```python
from build123d import *

# Parameters (mm, degrees)
BOSS_EXTRUDE1_DEPTH = 25.4
SKETCH2_R           = 14.2875
CUT_EXTRUDE1_DEPTH  = 83.854726027
SKETCH3_W           = 50.8
SKETCH3_H           = 38.1
CUT_EXTRUDE3_DEPTH  = 9.525
SKETCH4_W           = 11.43
SKETCH4_H           = 12.7
BOSS_EXTRUDE2_DEPTH = 38.1
CHAMFER1_SIZE       = 6.35
SKETCH5_W           = 6.35
SKETCH5_H           = 69.85
BOSS_EXTRUDE3_DEPTH = 95.25
SKETCH7_R           = 6.35
CUT_EXTRUDE5_DEPTH  = 145.139405178
SKETCH8_W           = 38.1
SKETCH8_H           = 9.525
CUT_EXTRUDE6_DEPTH  = 9.525
CHAMFER4_SIZE       = 9.525
SKETCH10_W          = 50.8
SKETCH10_H          = 72.641150816
BOSS_EXTRUDE5_DEPTH = 6.35
BOSS_EXTRUDE9_DEPTH = 50.8
SKETCH13_W          = 38.1
SKETCH13_H          = 50.8
CUT_EXTRUDE8_DEPTH  = 6.3754
SKETCH14_R          = 2.4892
CUT_EXTRUDE9_DEPTH  = 19.05
SKETCH15_R          = 2.4892
CUT_EXTRUDE10_DEPTH = 19.0246


with BuildPart() as part:
    # Sketch1 → Boss-Extrude1 (new, symmetric)
    with BuildSketch(Plane.XY):
        Polygon((-25.4, -47.625), (-19.05, -47.625), (-19.05, -9.525), (19.05, -9.525), (19.05, -47.625), (25.4, -47.625), (25.4, 60.325), (19.05, 60.325), (19.05, 9.525), (-19.05, 9.525), (-19.05, 60.325), (-25.4, 60.325), align=None)
    extrude(amount=BOSS_EXTRUDE1_DEPTH, both=True)

    # Sketch2 → Cut-Extrude1 (cut, through all)
    with BuildSketch(Plane.ZY.offset(25.4)):
        with Locations(Location((0, 34.925, 0), (0, 0, 270))):
            Circle(SKETCH2_R)
    extrude(amount=-CUT_EXTRUDE1_DEPTH, mode=Mode.SUBTRACT)

    # Sketch3 → Cut-Extrude3 (cut)
    with BuildSketch(Plane(origin=(0, 0, 25.4), x_dir=(-1, 0, 0), z_dir=(0, 0, -1))):
        with Locations((0, -28.575)):
            Rectangle(SKETCH3_W, SKETCH3_H)
    extrude(amount=CUT_EXTRUDE3_DEPTH, mode=Mode.SUBTRACT)

    # Sketch4 → Boss-Extrude2 (add)
    with BuildSketch(Plane.ZY.offset(-19.05)):
        with Locations((-19.685, 53.975)):
            Rectangle(SKETCH4_W, SKETCH4_H)
    extrude(amount=BOSS_EXTRUDE2_DEPTH)

    # Chamfer1
    chamfer1_edges = [part.edges().sort_by_distance(p)[0] for p in [
        (0, 60.325, -25.4),
    ]]
    chamfer(chamfer1_edges, length=CHAMFER1_SIZE)

    # Sketch5 → Boss-Extrude3 (add)
    with BuildSketch(Plane.XY.offset(25.4)):
        with Locations((-22.225, 25.4)):
            Rectangle(SKETCH5_W, SKETCH5_H)
        with Locations((22.225, 25.4)):
            Rectangle(SKETCH5_W, SKETCH5_H)
    extrude(amount=BOSS_EXTRUDE3_DEPTH)

    # Sketch7 → Cut-Extrude5 (cut, through all)
    with BuildSketch(Plane.ZY.offset(25.4)):
        with Locations(Location((38.1, 6.35, 0), (0, 0, 270))):
            Circle(SKETCH7_R)
    extrude(amount=-CUT_EXTRUDE5_DEPTH, mode=Mode.SUBTRACT)

    # Sketch8 → Cut-Extrude6 (cut)
    with BuildSketch(Plane.XY.offset(25.4)):
        with Locations((0, 4.7625)):
            Rectangle(SKETCH8_W, SKETCH8_H)
    extrude(amount=-CUT_EXTRUDE6_DEPTH, mode=Mode.SUBTRACT)

    # Chamfer4
    chamfer4_edges = [part.edges().sort_by_distance(p)[0] for p in [
        (0, 0, 25.4),
    ]]
    chamfer(chamfer4_edges, length=CHAMFER4_SIZE - 0.0001)  # a hair under: the kernel refuses the full size

    # Sketch10 → Boss-Extrude5 (add)
    with BuildSketch(Plane.XZ.offset(9.525)):
        with Locations((0, 84.329424592)):
            Rectangle(SKETCH10_W, SKETCH10_H)
    extrude(amount=BOSS_EXTRUDE5_DEPTH)

    # Sketch12 → Boss-Extrude9 (add)
    with BuildSketch(Plane.XY.offset(120.65)):
        Polygon((-25.4, 60.325), (-19.05, 60.325), (-19.05, 9.525), (19.05, 9.525), (19.05, 60.325), (25.4, 60.325), (25.4, -47.625), (19.05, -47.625), (19.05, -15.875), (-19.05, -15.875), (-19.05, -47.625), (-25.4, -47.625), align=None)
    extrude(amount=BOSS_EXTRUDE9_DEPTH)

    # Sketch13 → Cut-Extrude8 (cut)
    with BuildSketch(Plane(origin=(0, -15.875, 0), x_dir=(-1, 0, 0), z_dir=(0, -1, 0))):
        with Locations((0, -146.05)):
            Rectangle(SKETCH13_W, SKETCH13_H)
    extrude(amount=-CUT_EXTRUDE8_DEPTH, mode=Mode.SUBTRACT)

    # Sketch14 → Cut-Extrude9 (cut)
    with BuildSketch(Plane.XZ.offset(9.525)):
        with Locations(Location((0, -19.05, 0), (0, 0, 270))):
            Circle(SKETCH14_R)
        with Locations(Location((0, 6.35, 0), (0, 0, 270))):
            Circle(SKETCH14_R)
    extrude(amount=-CUT_EXTRUDE9_DEPTH, mode=Mode.SUBTRACT)

    # Sketch15 → Cut-Extrude10 (cut)
    with BuildSketch(Plane.XZ.offset(9.4996)):
        with Locations(Location((0, 158.75, 0), (0, 0, 270))):
            Circle(SKETCH15_R)
        with Locations(Location((0, 133.35, 0), (0, 0, 270))):
            Circle(SKETCH15_R)
    extrude(amount=-CUT_EXTRUDE10_DEPTH, mode=Mode.SUBTRACT)


solid = part.part
```
Geometry check sheet. Reference: the model listing, model coordinates, mm. A direction names the side the tool comes from. Coordinates: 2 decimals unless noted, no trailing zeros. Write each loop counter-clockwise with the first axis right and the second up, starting at its lowest first coordinate (ties: lowest second). Pieces come first, ordered by that corner, then holes. Notation, with made-up numbers: M 34.5,37 L 69.5,37 A13 cw 69.5,47 Z; hole C -15,73.5 d8. An arc over 180 degrees is marked long. Use one line per item in the form item = value. Start each with the question number.
1) Set-up check for faces 1 (the flat face through (19.05, -28, -4)), 2 (the flat face through (19.05, 19, 96)), 3 (the flat face through (0, 9.525, 146)), 4 (the flat face through (22, -32, 120.65)), 5 (the flat face through (-0.267, -4.696, 20.571)): record each of +Z, -Z, +X, -X, +Y, -Y from which the full face is reachable in a straight line by a thin tool's end or side.
2) Section check A-A on x = -12. State how many separate pieces and enclosed holes the cut face has, and give its area (3 significant figures).
3) Go/stop test with flat-tipped pins: pin 1 Ø1.9 at (x, y) = (-12.5, -14) entering from -Z; pin 2 Ø2 at (x, z) = (7.5, 139) entering from -Y. Record where each tip stops, or that it passes through.
4) Thickness scan on probe 1 along X at (y, z) = (28, 91.5); probe 2 along Y at (x, z) = (12.5, -14.5) (3 decimals); probe 3 along Z at (x, y) = (-22, 6). Record the ranges inside material, lowest first. Write a range as from..to.
5) Section check D-D on y = -19. Enter the section's corners in (x, z) (3 decimals), and give its area (3 significant figures).
6) Section check B-B on z = 133.35. Enter the section's corners in (x, y) (3 decimals).
7) Section check C-C on y = 18.5. Enter the section's corners in (x, z), and give its area (3 significant figures).
8) Release check for a two-part mould opening along Z. For faces 6 (the flat face through (-22, -28, 15.875)), 7 (the flat face through (-21, 60.325, 62)), 8 (the flat face through (0, -13, 120.65)) record: pulls with the +Z half, pulls with the -Z half, needs draft (parallel to the pull), parting line crosses it, or undercut.
Responses:
q1.face_1 = -Z, -Y
q1.face_2 = none
q1.face_3 = +Z, -Z, +Y
q1.face_4 = +X, -X, -Y
q1.face_5 = +Y
q2.separate_pieces = 4
q2.enclosed_holes = 0
q2.area = 2,380 mm2
q3.pin_1 = 48.01
q3.pin_2 = -9.5
q4.probe_1 = -25.4..-19.05, 19.05..25.4
q4.probe_2 = -9.525..9.525, 47.625..60.325
q4.probe_3 = -25.4..31.76, 44.44..171.45
q5.outline = M -25.4,-25.4 L -19.05,-25.4 L -19.05,15.875 L -25.4,15.875 Z; M -25.4,120.65 L -19.05,120.65 L -19.05,171.45 L -25.4,171.45 Z; M 19.05,-25.4 L 25.4,-25.4 L 25.4,15.875 L 19.05,15.875 Z; M 19.05,120.65 L 25.4,120.65 L 25.4,171.45 L 19.05,171.45 Z
q5.area = 1,170 mm2
q6.outline = M -25.4,-47.625 L -19.05,-47.625 L -19.05,-9.5 L -2.489,-9.5 L -2.489,9.525 L -19.05,9.525 L -19.05,60.325 L -25.4,60.325 Z; M 2.489,-9.5 L 19.05,-9.5 L 19.05,-47.625 L 25.4,-47.625 L 25.4,60.325 L 19.05,60.325 L 19.05,9.525 L 2.489,9.525 Z
q7.outline = M -25.4,-25.4 L -19.05,-25.4 L -19.05,171.45 L -25.4,171.45 Z; M 19.05,-25.4 L 25.4,-25.4 L 25.4,171.45 L 19.05,171.45 Z
q7.area = 2,500 mm2
q8.face_6 = undercut
q8.face_7 = needs draft
q8.face_8 = pulls with the +Z half
